Can you work these out from the model? Positions are in its coordinate system, mm. Give positions to 0.01 mm unless a question says otherwise; leave off trailing zeros. Write each loop counter-clockwise with the first axis right and the second up, starting at its lowest first coordinate (ties: lowest second). Pieces come first, ordered by that corner, then holes. Notation, with made-up numbers: M -3.75,-1.5 L 7.25,-1.5 A27 ccw 7.25,22.5 Z; hole C -2,-29 d2. An arc over 180 degrees is marked long. Write each question's results on one line, items separated by ' | '.
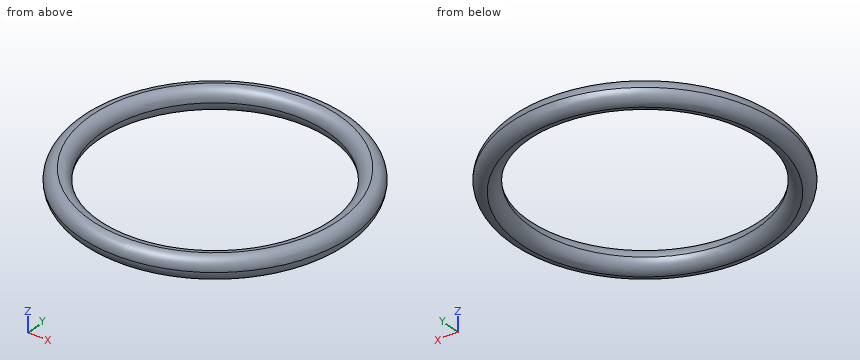
from build123d import *

# Parameters (mm, degrees)
F0_R     = 60
F0_R_2   = 50
F1_DEPTH = 10
F2_R     = 4.99999


# Not quite as in the source:
# - a fillet or chamfer is up to 0.001 mm smaller than in the source, because OpenCascade refuses the exact size


with BuildPart() as f1:
    # F0 (on Top) → F1 (new body)
    with BuildSketch(Plane.XY):
        with Locations((-48.8860793412, 39.2916202545)):
            Circle(F0_R)
        with Locations((-48.8860793412, 39.2916202545)):
            Circle(F0_R_2, mode=Mode.SUBTRACT)
    extrude(amount=F1_DEPTH)

    # F2 (radius 5 in the source; OpenCascade refuses exactly that, so slightly less here)
    f2_edges = [f1.edges().sort_by_distance(p)[0] for p in [
        (-108.886079, 39.29162, 10),
        (-108.886079, 39.29162, 0),
        (-98.886079, 39.29162, 10),
        (-98.886079, 39.29162, 0),
    ]]
    fillet(f2_edges, radius=F2_R)


solid = f1.part
Item 1: I want a section at A-A, the plane z = 2.5. Please give me the cut outline in (x, y), and give its area (3 significant figures).
Geometry says:
outline: C -48.89,39.29 d118.66; hole C -48.89,39.29 d101.34 | area: 2,990 mm2
Item 2: I'm going to push flat-ended pins straight in: pin 1 (5 mm diameter, centred on x = -1.5, y = 5.5, fed in from +Z); pin 2 (2 mm diameter, centred on y = 63.5, z = 3, fed in from +X); pin 3 (6 mm diameter, centred on y = 52, z = 4.5, fed in from +X). Where does each tip first touch, or does it pass through?
Geometry says:
pin 1: stops at z = 9.95 | pin 2: stops at x = 6.14 | pin 3: stops at x = 10.32
Item 3: I want a section at B-B, the plane z = 8.5. Please give me the cut outline in (x, y).
Geometry says:
outline: C -48.89,39.29 d117.14; hole C -48.89,39.29 d102.86
Item 4: If I drill on line 1 (X direction, y = 37, z = 5); line 2 (Y direction, x = -13, z = 1.5); line 3 (Y direction, x = -63.5, z = 3.75), over which ranges is the centre line in solid material (lowest first)? Write a range as from..to.
Geometry says:
line 1: x = -108.84..-98.83, 1.06..11.07 | line 2: y = -7..2.45, 76.13..85.58 | line 3: y = -18.74..-8.69, 87.27..97.32
